from build123d import *

# Parameters (mm, degrees)
F0_W     = 55.88
F0_H     = 55.88
F1_DEPTH = 88.9
F2_T     = -5.08
F3_R     = 23.8404105374
F4_DEPTH = 88.9


with BuildPart() as f1:
    # F0 (on Top) → F1 (new body)
    with BuildSketch(Plane.XY):
        Rectangle(F0_W, F0_H)
    extrude(amount=F1_DEPTH)

    # F2 (hollow: no face is removed)
    offset(amount=F2_T, mode=Mode.SUBTRACT)

    # F3 (on Top) → F4 (cut)
    with BuildSketch(Plane.XY):
        Circle(F3_R)
    extrude(amount=F4_DEPTH, mode=Mode.SUBTRACT)


solid = f1.part
Input: part model. Units: mm. Frame: model coordinates. A direction names the side the tool comes from. Give positions to 0.01 mm unless a question says otherwise; leave off trailing zeros. Order: outer loops, then holes, each group sorted by start corner. A loop starts at its lowest first (then second) coordinate and runs counter-clockwise, first axis right, second up. Notation, with made-up numbers: (87, 72.5) -> (119, 72.5) arc R28 cw to (119, 90.5) -> close; hole circle Ø2 at (67, 32.5). An arc over 180 degrees is marked (long way). Use one line per item in the form item = value.
1) Mould query, pull axis X, two halves, no side actions, for faces 3 (the flat face through (-18, -18, 5.08)), 4 (the flat face through (-27.94, 0, 44)), 5 (the flat face through (27.94, 0, 44)). Classes: pulls with the +X half, pulls with the -X half, needs draft (parallel to the pull), parting line crosses it, or undercut.
Response values:
face_3 = undercut
face_4 = pulls with the -X half
face_5 = pulls with the +X half
2) First-contact query: pin 1 Ø13 at (x, y) = (-17.5, 11.5) entering from -Z; pin 2 Ø12 at (x, y) = (1.5, 14) entering from +Z. Flat tips, straight axial feed; report the tip coordinate or a pass-through.
Response values:
pin_1 = 0
pin_2 = through
3) Line query: probe 1 along X at (y, z) = (-15.5, 12.5); probe 2 along Y at (x, z) = (0, 45). Output: solid intervals per line, ascending.
Response values:
probe_1 = -27.94 to -22.86, 22.86 to 27.94
probe_2 = -27.94 to -23.84, 23.84 to 27.94
4) Section D-D, the plane y = -18.5. Return loops of the section in (x, z).
Response values:
outline = (-27.94, 0) -> (-15.04, 0) -> (-15.04, 5.08) -> (-22.86, 5.08) -> (-22.86, 83.82) -> (-15.04, 83.82) -> (-15.04, 88.9) -> (-27.94, 88.9) -> close; (15.04, 0) -> (27.94, 0) -> (27.94, 88.9) -> (15.04, 88.9) -> (15.04, 83.82) -> (22.86, 83.82) -> (22.86, 5.08) -> (15.04, 5.08) -> close
5) Reachability of faces 1 (the flat face through (24, 0, 88.9)), 2 (the flat face through (22.86, -15, 44)) from +Z, -Z, +X, -X, +Y, -Y: full face, straight path, thin tool, end or side. Return the list, or none.
Response values:
face_1 = +Z, +X, -X, +Y, -Y
face_2 = none
6) Section B-B, the plane y = 0. Return loops of the section in (x, z), and give its area (3 significant figures).
Response values:
outline = (-27.94, 0) -> (-23.84, 0) -> (-23.84, 88.9) -> (-27.94, 88.9) -> close; (23.84, 0) -> (27.94, 0) -> (27.94, 88.9) -> (23.84, 88.9) -> close
area = 729 mm^2
7) Section A-A, the plane z = 9. Return loops of the section in (x, y), and give its area (3 significant figures).
Response values:
outline = (-27.94, -27.94) -> (27.94, -27.94) -> (27.94, 27.94) -> (-27.94, 27.94) -> close; hole (-22.86, -22.86) -> (-6.77, -22.86) arc R23.84 ccw to (6.77, -22.86) -> (22.86, -22.86) -> (22.86, -6.77) arc R23.84 ccw to (22.86, 6.77) -> (22.86, 22.86) -> (6.77, 22.86) arc R23.84 ccw to (-6.77, 22.86) -> (-22.86, 22.86) -> (-22.86, 6.77) arc R23.84 ccw to (-22.86, -6.77) -> close
area = 997 mm^2
